Autodesk Inventor part; units mm, degrees
ref_plane "YZ Plane" through (0, 0, 0) normal (1, 0, 0) x (0, 1, 0)
ref_plane "XZ Plane" through (0, 0, 0) normal (0, 1, 0) x (-1, 0, 0)
ref_plane "XY Plane" through (0, 0, 0) normal (0, 0, 1) x (1, 0, 0)
sketch "Sketch1" plane through (0, 0, 0) normal (0, 0, 1) x (1, 0, 0)
  circle A0 centre (0, 9.4768) radius 4.1
  circle A1 centre (0, 9.4768) radius 11.1
  arc A2 (5.7519, 50.2372) -> (4.0065, 45.5517) centre (13.9526, 44.5146) ccw
  arc A3 (-3.9935, 45.5517) -> (-5.7388, 50.2372) centre (-13.9395, 44.5146) ccw
  line L0 (4.0065, 55.0581) -> (4.0065, 33.0581)
  line L1 (-3.9935, 33.0581) -> (-3.9935, 55.0581)
  line L2 (-3.9935, 55.0581) -> (4.0065, 55.0581)
  line L3 (0.0065, 55.0581) -> (5.7519, 50.2372)
  line L4 (0.0065, 55.0581) -> (0.0065, 47.5581) construction
  line L5 (0.0065, 55.0581) -> (-5.7388, 50.2372)
  circle A4 centre (0.0065, 55.0581) radius 7.5
  line L6 (4.0065, 33.0581) -> (-3.9935, 33.0581)
  line L7 (0.0065, 55.0581) -> (0.0065, 32.0581) construction
  line L8 (4.0065, 55.0581) -> (4.0065, 32.0581)
  line L9 (-3.9935, 32.0581) -> (-3.9935, 55.0581)
  arc A5 (4.0065, 55.0581) -> (-3.9935, 55.0581) centre (0.0065, 55.0581) ccw
  arc A6 (-3.9935, 32.0581) -> (4.0065, 32.0581) centre (0.0065, 32.0581) ccw
  line L10 (-15.9677, -6.0429) -> (18.5773, -6.0429)
  line L11 (18.5773, -6.0429) -> (18.5773, 65.522)
  line L12 (18.5773, 65.522) -> (-15.9677, 65.522)
  line L13 (-15.9677, 65.522) -> (-15.9677, -6.0429)
  point P0 (0, 0)
  point P1 (0.0065, 55.0581)
  point P2 (0.0065, 55.0581)
  point P3 (0.0065, 43.5581)
  point P4 (-3.9935, 45.5517)
  dimension "d2" = 15
  dimension "d0" = 8.2
  dimension "d1" = 22.2
  dimension "d3" = 22
  dimension "d4" = 8
  dimension "d5" = 50
  dimension "d6" = 5
  dimension "d7" = 10
  dimension "d8" = 23
extrude "Extrusion1" add sketch "Sketch1" along normal blind 3 contours A1 | L13 L12 L11 L10
extrude "Extrusion2" add sketch "Sketch1" against normal blind 8 contours L13 L12 L11 L10
properties part number "Prueba3D"
CAD build for the part. Positions are in the model's coordinates, mm. A direction names the side the tool comes from. Coordinates: 2 decimals unless noted, no trailing zeros. Loops run counter-clockwise (first coordinate to the right, second up) from the corner with the lowest first, then second, coordinate; pieces in that order, holes last. Notation, with made-up numbers: (36, -25.5) - (84, -25.5) arc R19 cw to (84, -6.5) - close; hole circle Ø2 at (-9.5, -28.75). An arc over 180 degrees is marked (long way). Return JSON: item names as keys, results as strings.
1. Drop flat-ended pins along their axis: pin 1 (12 mm diameter, centred on x = 0.01, y = 55.06, fed in from +Z); pin 2 (18 mm diameter, centred on x = 0, y = 9.48, fed in from -Z). Give the stop position or say it passes through.
Result:
{"pin 1": "passes through", "pin 2": "stops at z = 0"}
2. Mould opens along X. For faces 4 (the flat face through (-3.994, 39, -2)), 5 (the flat face through (2, 65.522, -2)), 6 (the flat face through (18.577, 29, -2)) say: released by +X, released by -X, zero draft, split by the parting line, or undercut.
Result:
{"face 4": "undercut", "face 5": "zero draft", "face 6": "released by +X"}
3. Probe L1, parallel to Y at x = 0, z = 2.4; L2, parallel to X at y = 34.5, z = 2; L3, parallel to Z at x = -4.5, y = 14. List the from-to ranges inside material, lowest first. Write a range as from..to.
Result:
{"L1": "y = -6.04..5.38, 13.58..28.06, 62.56..65.52", "L2": "x = -15.97..-3.99, 4.01..18.58", "L3": "z = 0..3"}
4. Band-saw the part on C-C (z = -5.75). Give the cut face in (x, y), and give its area (3 significant figures).
Result:
{"outline": "(-15.97, -6.04) - (18.58, -6.04) - (18.58, 65.52) - (-15.97, 65.52) - close; hole circle Ø22.2 at (0, 9.48); hole (-5.74, 50.24) arc R10 cw to (-3.99, 45.55) - (-3.99, 32.06) arc R4 ccw to (4.01, 32.06) - (4.01, 45.55) arc R10 cw to (5.75, 50.24) arc R7.5 ccw (long way) to start", "area": "1,750 mm2"}
5. Band-saw the part on B-B (y = 54). Give the cut face in (x, z).
Result:
{"outline": "(-15.97, -8) - (-7.42, -8) - (-7.42, 3) - (-15.97, 3) - close; (7.43, -8) - (18.58, -8) - (18.58, 3) - (7.43, 3) - close"}
6. Band-saw the part on A-A (x = 0). Give the cut face in (y, z).
Result:
{"outline": "(-6.04, -8) - (-1.62, -8) - (-1.62, 0) - (5.38, 0) - (5.38, 3) - (-6.04, 3) - close; (13.58, 0) - (20.58, 0) - (20.58, -8) - (28.06, -8) - (28.06, 3) - (13.58, 3) - close; (62.56, -8) - (65.52, -8) - (65.52, 3) - (62.56, 3) - close"}
7. Band-saw the part on D-D (x = -6.5). Give the cut face in (y, z).
Result:
{"outline": "(-6.04, -8) - (0.48, -8) - (0.48, 0) - (18.47, 0) - (18.47, -8) - (51.33, -8) - (51.33, 3) - (-6.04, 3) - close; (58.79, -8) - (65.52, -8) - (65.52, 3) - (58.79, 3) - close"}
8. 3-axis set-ups, long thin cutter, end or side, ignore diameter. For faces 1 (the flat face through (5, 30, -8)), 2 (the cylindrical face through (4.594, 48.038, -2.423)), 3 (the cylindrical face through (-2.41, -1.36, -3.94)): which of +Z, -Z, +X, -X, +Y, -Y reach the whole face in a straight line?
Result:
{"face 1": "-Z, +X, -X, +Y, -Y", "face 2": "+Z, -Z", "face 3": "-Z"}
